from build123d import *

# Parameters (mm, degrees)
EXTRUDE_1_DEPTH     = 26
SKETCH_2_R          = 4.25
CUT_EXTRUDE_1_DEPTH = 5
SKETCH_3_R          = 4.25
CUT_EXTRUDE_2_DEPTH = 5
FILLET_1_R          = 4
FILLET_2_R          = 1


with BuildPart() as part:
    # Эскиз1 → Бобышка-Вытянуть1 (new body, symmetric)
    with BuildSketch(Plane.XY):
        Polygon((0, 0), (-42.426406871, 42.426406871), (-38.890872965, 45.961940777), (-15.028558569, 22.099626381), (26.253591352, 5), (60, 5), (60, 0), align=None)
        Polygon((-14.313708499, 18.556349186), (23.242640687, 3), (1.242640687, 3), align=None, mode=Mode.SUBTRACT)
    extrude(amount=EXTRUDE_1_DEPTH, both=True)

    # Эскиз2 → Вырез-Вытянуть1 (cut)
    with BuildSketch(Plane(origin=(0, 0, 0), x_dir=(0, 0, 1), z_dir=(-0.707106781, -0.707106781, 0))):
        with Locations(Location((-15, 45, 0), (0, 0, 270))):  # turned: the seam where the file's is
            Circle(SKETCH_2_R)
        with Locations(Location((15, 45, 0), (0, 0, 270))):  # turned: the seam where the file's is
            Circle(SKETCH_2_R)
    extrude(amount=-CUT_EXTRUDE_1_DEPTH, mode=Mode.SUBTRACT)

    # Эскиз3 → Вырез-Вытянуть2 (cut)
    with BuildSketch(Plane.XZ):
        with Locations(Location((45, 15, 0), (0, 0, 270))):  # turned: the seam where the file's is
            Circle(SKETCH_3_R)
        with Locations(Location((45, -15, 0), (0, 0, 270))):  # turned: the seam where the file's is
            Circle(SKETCH_3_R)
    extrude(amount=-CUT_EXTRUDE_2_DEPTH, mode=Mode.SUBTRACT)

    # Скругление1
    fillet_1_edges = [part.edges().sort_by_distance(p)[0] for p in [
        (-38.890872965, 45.961940777, 0),
        (60, 5, 0),
    ]]
    fillet(fillet_1_edges, radius=FILLET_1_R)

    # Скругление2
    fillet_2_edges = [part.edges().sort_by_distance(p)[0] for p in [
        (-14.313708499, 18.556349186, 0),
        (1.242640687, 3, 0),
        (23.242640687, 3, 0),
    ]]
    fillet(fillet_2_edges, radius=FILLET_2_R)


solid = part.part
Could you check a few things on this model? Use its own coordinates, in mm. A direction names the side the tool comes from. Give positions to 0.01 mm unless a question says otherwise; leave off trailing zeros. Order: outer loops, then holes, each group sorted by start corner. A loop starts at its lowest first (then second) coordinate and runs counter-clockwise, first axis right, second up.
1. We'd pull the mould along Z, two halves only. Please class faces 1 (the cylindrical face through (-32.462, 35.948, 12.414)), 2 (the flat face through (-25.69, 32.76, 0.36)), 3 (the flat face through (5, 11, -26)): pulls with the +Z half, pulls with the -Z half, needs draft (parallel to the pull), parting line crosses it, or undercut.
2. I need wall thicknesses on L1, parallel to X at y = 4, z = 15; L2, parallel to X at y = 13, z = 16.5; L3, parallel to Y at x = -0.5, z = 5.5. Which ranges of each line are inside material? Lowest first, please.
3. Suppose I cut it at A-A (z = -13). List the corners of the cut face in (x, y) for me, plus the area to 3 significant figures.
4. Suppose I cut it at D-D (z = 3.5). List the corners of the cut face in (x, y) for me, plus the area to 3 significant figures.
5. Suppose I cut it at B-B (x = 45). List the corners of the cut face in (y, z) for me.
6. For faces 4 (the flat face through (41, 5, 0)), 5 (the flat face through (30, 0, 0)), 6 (the flat face through (4.27, 10.86, 0.36)), which set-ups out of +Z, -Z, +X, -X, +Y, -Y let a thin tool reach every point of the face, with its end or its side?
7. Will these pins go through, and if not, where does the flat tip stop? P1, Ø4, axis at x = -18, z = -10.5, coming from the -Y side; P2, Ø4, axis at y = 13, z = -2, coming from the +X side; P3, Ø5, axis at y = 23, z = -2, coming from the -X side.
8. Suppose I cut it at C-C (y = 12). List the corners of the cut face in (x, z) for me.
Solved:
1. face 1: undercut
1. face 2: needs draft
1. face 3: pulls with the -Z half
2. L1: x = -4 to 0.24, 19.22 to 40.75, 49.25 to 58.65
2. L2: x = -13 to -8.76, -0.9 to 6.94
2. L3: y = 0.5 to 4.74, 12.83 to 16.08
3. outline: (-42.43, 42.43) - (-34.47, 34.47) - (-30.94, 38.01) - (-36.06, 43.13) arc R4 ccw to (-41.72, 43.13) - close; (-29.17, 29.17) - (0, 0) - (41.25, 0) - (41.25, 5) - (26.25, 5) - (-15.03, 22.1) - (-25.63, 32.7) - close; (48.75, 0) - (60, 0) - (60, 1) arc R4 ccw to (56, 5) - (48.75, 5) - close; hole (-10.76, 15) - (0.95, 3.29) arc R1 ccw to (1.66, 3) - (18.22, 3) arc R1 ccw to (18.6, 4.92) - (-9.67, 16.63) arc R1 ccw to start
3. area: 551 mm2
4. outline: (-42.43, 42.43) - (0, 0) - (60, 0) - (60, 1) arc R4 ccw to (56, 5) - (26.25, 5) - (-15.03, 22.1) - (-36.06, 43.13) arc R4 ccw to (-41.72, 43.13) - close; hole (-10.76, 15) - (0.95, 3.29) arc R1 ccw to (1.66, 3) - (18.22, 3) arc R1 ccw to (18.6, 4.92) - (-9.67, 16.63) arc R1 ccw to start
4. area: 626 mm2
5. outline: (0, -26) - (5, -26) - (5, -19.25) - (0, -19.25) - close; (0, -10.75) - (5, -10.75) - (5, 10.75) - (0, 10.75) - close; (0, 19.25) - (5, 19.25) - (5, 26) - (0, 26) - close
6. face 4: +Z, -Z, +X, +Y
6. face 5: +Z, -Z, +X, -X, -Y
6. face 6: +Z, -Z
7. P1: stops at y = 16
7. P2: stops at x = 11.77
7. P3: stops at x = -25.5
8. outline: (-12, -26) - (-7.76, -26) - (-7.76, 26) - (-12, 26) - close; (1.51, -26) - (9.35, -26) - (9.35, 26) - (1.51, 26) - close
